from build123d import *

# Parameters (mm, degrees)
EXTRUDE_1_DEPTH          = 64
EXTRUDE_2_DEPTH          = 60
SKETCH_1_4_R             = 7.5
EXTRUDE_3_DEPTH          = 12
FILLET_1_R               = 15
CUT_EXTRUDE_1_DEPTH      = 117.365802537
CUT_EXTRUDE_1_DEPTH_BACK = 117.365802537
SKETCH_3_R               = 7.5
CUT_EXTRUDE_START        = -48
CUT_EXTRUDE_2_DEPTH      = 32
SKETCH_5_R               = 8
CUT_EXTRUDE_3_DEPTH      = 108.275346655


with BuildPart() as part:
    # Sketch 1 → Extrude 1 (new body)
    with BuildSketch(Plane.XY):
        with BuildLine():
            Line((25, 0), (50, 0))
            ThreePointArc((50, 0), (0, 50), (-50, 0))
            Line((-50, 0), (-25, 0))
            ThreePointArc((-25, 0), (0, 25), (25, 0))
        make_face()
    extrude(amount=EXTRUDE_1_DEPTH)

    # Sketch 1_3 → Extrude 2 (add)
    with BuildSketch(Plane.XY):
        with BuildLine():
            Line((-74, 14), (-74, 0))
            Line((-74, 0), (-50, 0))
            ThreePointArc((-50, 0), (-49.497474683, 7.071067812), (-48, 14))
            Line((-48, 14), (-74, 14))
        make_face()
        with BuildLine():
            ThreePointArc((48, 14), (49.497474683, 7.071067812), (50, 0))
            Line((50, 0), (74, 0))
            Line((74, 0), (74, 14))
            Line((74, 14), (48, 14))
        make_face()
    extrude(amount=EXTRUDE_2_DEPTH)

    # Sketch 1_4 → Extrude 3 (add)
    with BuildSketch(Plane.XY):
        with BuildLine():
            Line((-15, 62), (-15, 47.696960071))
            ThreePointArc((-15, 47.696960071), (0, 50), (15, 47.696960071))
            Line((15, 47.696960071), (15, 62))
            ThreePointArc((15, 62), (0, 77), (-15, 62))
        make_face()
        with Locations((0, 62)):
            Circle(SKETCH_1_4_R, mode=Mode.SUBTRACT)
    extrude(amount=EXTRUDE_3_DEPTH)

    # Fillet 1
    fillet_1_edges = [part.edges().sort_by_distance(p)[0] for p in [
        (-74, 7, 60),
        (-74, 7, 0),
        (74, 7, 0),
        (74, 7, 60),
    ]]
    fillet(fillet_1_edges, radius=FILLET_1_R)

    # Sketch 3 → Cut-Extrude 1 (cut, two sides: drawn at the far end of the back side and taken through both)
    with BuildSketch(Plane(origin=(0, 14, 0), x_dir=(1, 0, 0), z_dir=(0, 1, 0)).offset(-CUT_EXTRUDE_1_DEPTH_BACK)):
        with Locations(Location((-59, -15, 0), (0, 0, 270))):
            Circle(SKETCH_3_R)
        with Locations(Location((-59, -45, 0), (0, 0, 270))):
            Circle(SKETCH_3_R)
        with Locations(Location((59, -15, 0), (0, 0, 90))):
            Circle(SKETCH_3_R)
        with Locations(Location((59, -45, 0), (0, 0, 270))):
            Circle(SKETCH_3_R)
    extrude(amount=CUT_EXTRUDE_1_DEPTH + CUT_EXTRUDE_1_DEPTH_BACK, mode=Mode.SUBTRACT)

    # Sketch 4 → Cut-Extrude 2 (cut)
    with BuildSketch(Plane.XY.offset(64).offset(CUT_EXTRUDE_START)):
        with BuildLine():
            Line((-23.748684174, 44), (23.748684174, 44))
            ThreePointArc((23.748684174, 44), (0, 50), (-23.748684174, 44))
        make_face()
    extrude(amount=CUT_EXTRUDE_2_DEPTH, mode=Mode.SUBTRACT)

    # Sketch 5 → Cut-Extrude 3 (cut, through all)
    with BuildSketch(Plane(origin=(0, 44, 0), x_dir=(1, 0, 0), z_dir=(0, 1, 0))):
        with Locations(Location((0, -32, 0), (0, 0, 270))):
            Circle(SKETCH_5_R)
    extrude(amount=-CUT_EXTRUDE_3_DEPTH, mode=Mode.SUBTRACT)


solid = part.part
Design review of the part built by this model. Coordinates are the model's own, in mm. A direction names the side the tool comes from. Give positions to 0.01 mm unless a question says otherwise; leave off trailing zeros. Loops run counter-clockwise (first coordinate to the right, second up) from the corner with the lowest first, then second, coordinate; pieces in that order, holes last. Notation, with made-up numbers: (-10.5, 78) - (-1.5, 78) arc R25 ccw to (-1.5, 106) - close; hole circle Ø3 at (65.25, 77.5). An arc over 180 degrees is marked (long way). Use CSV: the item, a comma, the result in double quotes. Start each with the question number.
1. Add section A-A (x = -4). State the section outline as (y, z) points, plus the area to 3 significant figures.
2. Draft analysis for pull direction Z (two halves, no side actions). For faces 5 (the flat face through (0, 46, 16)), 6 (the flat face through (0, 46, 48)), 7 (the flat face through (-0.7, 25.4, 64)), 8 (the cylindrical face through (0, 77, 6)), state which applies: released by +Z, released by -Z, zero draft, split by the parting line, or undercut.
3. Machinability: for faces 1 (the flat face through (15, 55, 6)), 2 (the flat face through (-15, 55, 6)), 3 (the cylindrical face through (-9.065, 23.299, 31.552)), 4 (the flat face through (5, 44, 25)), which of the approach directions +Z, -Z, +X, -X, +Y, -Y give a long, thin tool a straight path to every point of the face, cutting with its end or side? Answer none if there is none.
4. Wall thickness on L1, parallel to Z at x = -59, y = 4.25; L2, parallel to X at y = 7.75, z = 15; L3, parallel to Y at x = 0, z = 2.5: over which ranges is each line inside the solid? List them lowest first.
5. Insertion check: P1, Ø8, axis at x = 60.5, z = 33.5, coming from the +Y side; P2, Ø12, axis at y = 48, z = 48.5, coming from the +X side; P3, Ø17, axis at x = 0, y = 62, coming from the +Z side; P4, Ø13.5, axis at x = 59, z = 45, coming from the -Y side. Each pin has a flat end and moves straight along its axis. Give the tip position at first contact, or say it passes through.
6. Add section C-C (z = 50). State the section outline as (x, y) points, plus the area to 3 significant figures.
7. Add section B-B (y = 66). State the section outline as (x, z) points, plus the area to 3 significant figures.
8. Add section D-D (y = 11). State the section outline as (x, z) points (3 decimals), plus the area to 3 significant figures.
Results found:
1,outline,"(24.68, 0) - (55.66, 0) - (55.66, 12) - (49.84, 12) - (49.84, 16) - (44, 16) - (44, 25.07) - (24.68, 25.07) - close; (24.68, 38.93) - (44, 38.93) - (44, 48) - (49.84, 48) - (49.84, 64) - (24.68, 64) - close; (68.34, 0) - (76.46, 0) - (76.46, 12) - (68.34, 12) - close"
1,area,"1,320 mm²"
2,face 5,"undercut"
2,face 6,"undercut"
2,face 7,"released by +Z"
2,face 8,"zero draft"
3,face 1,"+Z, -Z, +X, +Y"
3,face 2,"+Z, -Z, -X, +Y"
3,face 3,"+Z, -Z, -Y"
3,face 4,"+X, -X, +Y"
4,L1,"z = 0 to 7.5, 22.5 to 37.5, 52.5 to 60"
4,L2,"x = -74 to -66.5, -51.5 to -23.77, 23.77 to 51.5, 66.5 to 74"
4,L3,"y = 25 to 54.5, 69.5 to 77"
5,P1,"stops at y = 14"
5,P2,"stops at x = 27.13"
5,P3,"stops at z = 12"
5,P4,"passes through"
6,outline,"(-73.14, 0) - (-64.59, 0) - (-64.59, 14) - (-73.14, 14) - close; (-53.41, 0) - (-25, 0) arc R25 cw to (25, 0) - (53.41, 0) - (53.41, 14) - (48, 14) arc R50 ccw to (-48, 14) - (-53.41, 14) - close; (64.59, 0) - (73.14, 0) - (73.14, 14) - (64.59, 14) - close"
6,area,"3,300 mm²"
7,outline,"(-14.46, 0) - (-6.34, 0) - (-6.34, 12) - (-14.46, 12) - close; (6.34, 0) - (14.46, 0) - (14.46, 12) - (6.34, 12) - close"
7,area,"195 mm²"
8,outline,"(-74, 15) arc R15 ccw to (-59, 0) - (-22.45, 0) - (-22.45, 64) - (-48.775, 64) - (-48.775, 60) - (-59, 60) arc R15 ccw to (-74, 45) - close; (22.45, 0) - (59, 0) arc R15 ccw to (74, 15) - (74, 45) arc R15 ccw to (59, 60) - (48.775, 60) - (48.775, 64) - (22.45, 64) - close; hole circle Ø15 at (-59, 15); hole circle Ø15 at (-59, 45); hole circle Ø15 at (59, 15); hole circle Ø15 at (59, 45)"
8,area,"5,500 mm²"
